The figure shows three views and two pictorial views of one solid part (mm, origin at its lowest corner). Answer the questions. Coordinates: 2 decimals unless noted, no trailing zeros. Order: outer loops, then holes, each group sorted by start corner. A loop starts at its lowest first (then second) coordinate and runs counter-clockwise, first axis right, second up. Notation, with made-up numbers: M 61.5,23.5 L 117.5,23.5 A21 ccw 117.5,36.5 Z; hole C -30,64 d1. An arc over 180 degrees is marked long. Answer in a Markdown table with one row per item. Add a question column.
Item 1: The part is cut by section A-A (y = 91.44). Write down the section's boundary in (x, z) (1 decimal).
Item 2: The part is cut by section B-B (x = 66). Write down the section's boundary in (y, z) (1 decimal).
Item 3: The part is cut by section C-C (z = 1.15). State how many separate pieces and enclosed holes the cut face has, then the cut area to 3 significant figures.
Item 4: Consider line 1 (X direction, y = 96, z = 1.3) (1 decimal); line 2 (X direction, y = 139.7, z = 2.7) (1 decimal); line 3 (Y direction, x = 75, z = 0.25) (1 decimal). Determine where each line is inside the solid, lowest interval first. Write a range as from..to.
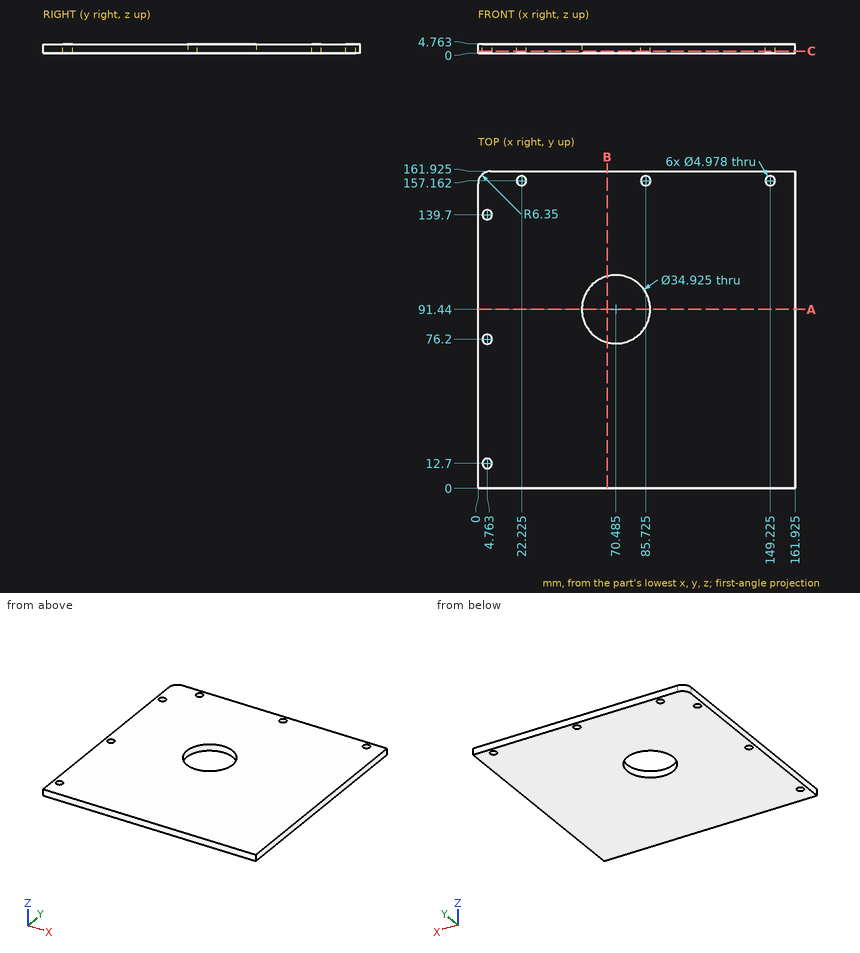
Reply:
| question | item | result |
|---|---|---|
| 1 | outline | M 0,0 L 53,0 L 53,4.8 L 0,4.8 Z; M 87.9,0 L 161.9,0 L 161.9,4.8 L 87.9,4.8 Z |
| 2 | outline | M 0,0 L 74.6,0 L 74.6,4.8 L 0,4.8 Z; M 108.3,0 L 161.9,0 L 161.9,4.8 L 108.3,4.8 Z |
| 3 | separate pieces | 1 |
| 3 | enclosed holes | 7 |
| 3 | area | 25,100 mm2 |
| 4 | line 1 | x = 0..53.6, 87.3..161.9 |
| 4 | line 2 | x = 0..2.3, 7.3..161.9 |
| 4 | line 3 | y = 0..74.6, 108.3..161.9 |
